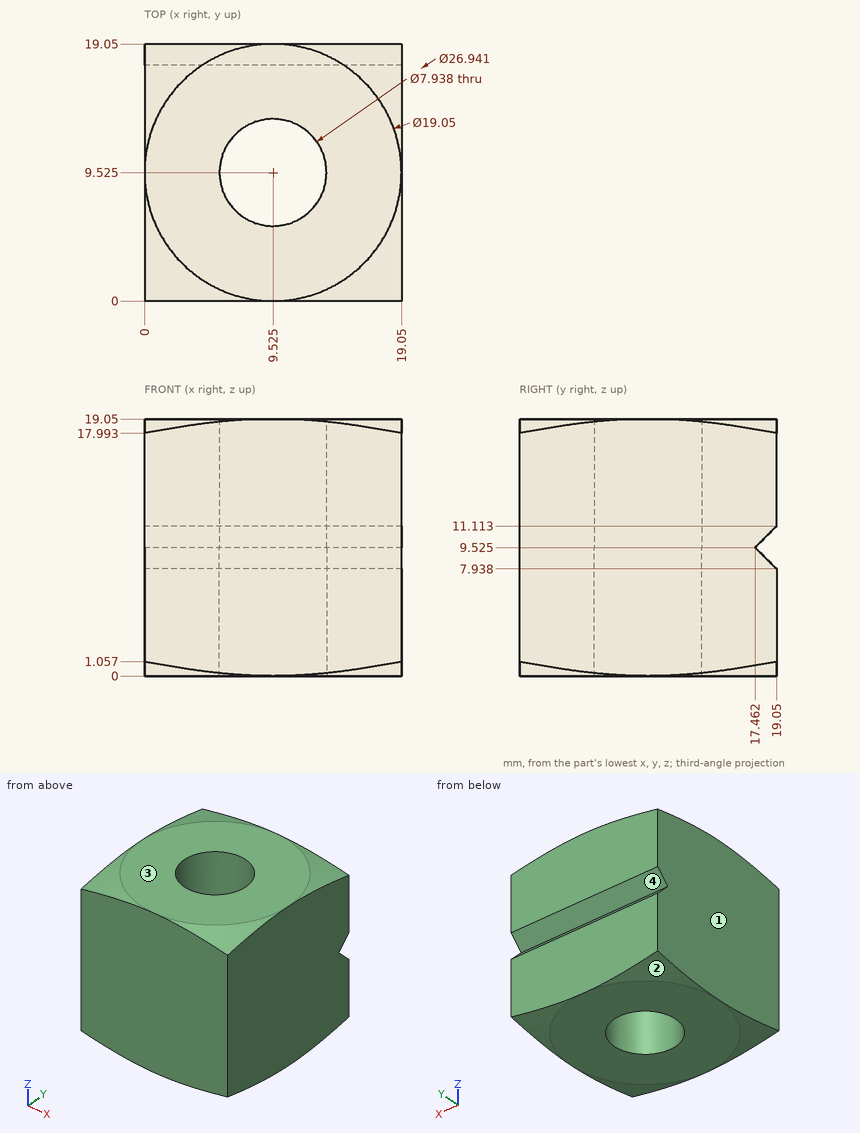
Can you work these out from the drawing? Everything is in mm from the part's minimum corner. Round coordinates to 2 decimals unless told otherwise and drop trailing zeros. Write each question's results on one line, items separated by ' | '. Start each with the question number.
1) Please list where these lines run through material, in increasing order: line 1 (X direction, y = 11.25, z = 11.5); line 2 (X direction, y = 11.75, z = 10.25); line 3 (Y direction, x = 8.75, z = 15).
2) We'd pull the mould along Z, two halves only. Please class the marked faces 1, 2, 3 and 4: released by +Z, released by -Z, zero draft, split by the parting line, or undercut.
3) For pin 1 Ø8 at (x, z) = (2, 2) entering from -Y, with a flat end and sliding along its axis, tell me the tip position at first contact or that it passes through.
Here are the results:
1) line 1: x = 0 to 5.95, 13.1 to 19.05 | line 2: x = 0 to 6.24, 12.81 to 19.05 | line 3: y = 0 to 5.63, 13.42 to 19.05
2) face 1: zero draft | face 2: released by -Z | face 3: released by +Z | face 4: undercut
3) pin 1: stops at y = 0
